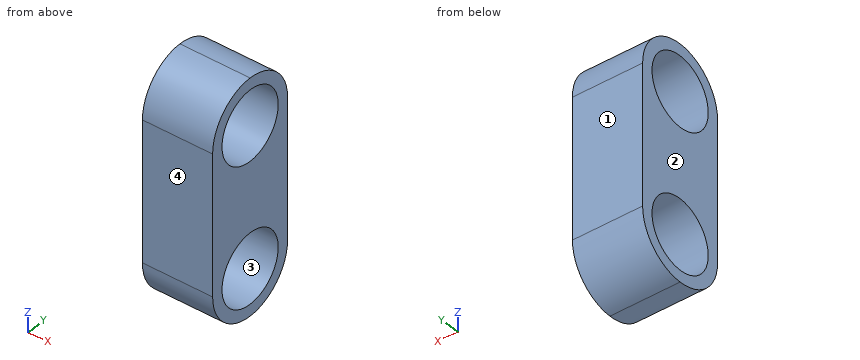
```python
from build123d import *

# Parameters (mm, degrees)
BOSS_EXTRUDE1_DEPTH = 3


with BuildPart() as part:
    # Sketch2 → Boss-Extrude1 (new body)
    with BuildSketch(Plane(origin=(0, 0, 0), x_dir=(0, 0, -1), z_dir=(1, 0, 0))):
        with BuildLine():
            Line((6, 0), (0, 0))
            ThreePointArc((0, 0), (1.414213562, -0.585786438), (2, -2))
            Line((2, -2), (4, -2))
            ThreePointArc((4, -2), (4.585786438, -0.585786438), (6, 0))
        make_face()
        with BuildLine():
            Line((4, -2), (2, -2))
            ThreePointArc((2, -2), (1.414213562, -3.414213562), (0, -4))
            Line((0, -4), (6, -4))
            ThreePointArc((6, -4), (4.585786438, -3.414213562), (4, -2))
        make_face()
        with BuildLine():
            ThreePointArc((2, -2), (1.414213562, -0.585786438), (0, 0))
            ThreePointArc((0, 0), (-1.414213562, -0.585786438), (-2, -2))
            Line((-2, -2), (-1.5, -2))
            ThreePointArc((-1.5, -2), (0, -0.5), (1.5, -2))
            Line((1.5, -2), (2, -2))
        make_face()
        with BuildLine():
            ThreePointArc((0, -4), (1.414213562, -3.414213562), (2, -2))
            Line((2, -2), (1.5, -2))
            ThreePointArc((1.5, -2), (0, -3.5), (-1.5, -2))
            Line((-1.5, -2), (-2, -2))
            ThreePointArc((-2, -2), (-1.414213562, -3.414213562), (0, -4))
        make_face()
        with BuildLine():
            ThreePointArc((8, -2), (7.414213562, -0.585786438), (6, 0))
            ThreePointArc((6, 0), (4.585786438, -0.585786438), (4, -2))
            Line((4, -2), (4.5, -2))
            ThreePointArc((4.5, -2), (6, -0.5), (7.5, -2))
            Line((7.5, -2), (8, -2))
        make_face()
        with BuildLine():
            ThreePointArc((6, -4), (7.414213562, -3.414213562), (8, -2))
            Line((8, -2), (7.5, -2))
            ThreePointArc((7.5, -2), (6, -3.5), (4.5, -2))
            Line((4.5, -2), (4, -2))
            ThreePointArc((4, -2), (4.585786438, -3.414213562), (6, -4))
        make_face()
    extrude(amount=BOSS_EXTRUDE1_DEPTH)


solid = part.part
```
Check sheet for the modelled part. Datum: model origin and axes. Units: mm. Face numbers are marked on the shaded views. Round coordinates to 2 decimals unless told otherwise and drop trailing zeros. Loops run counter-clockwise (first coordinate to the right, second up) from the corner with the lowest first, then second, coordinate; pieces in that order, holes last. Notation, with made-up numbers: (-9, 2) - (12, 2) arc R27 cw to (12, 18) - close; hole circle Ø11 at (81.25, 39.25). An arc over 180 degrees is marked (long way). Write item = value, one per line. Start each with the question number.
Q1. Depth check by flat-ended pin: P1, Ø1.5, axis at x = 2.5, y = -3.5, coming from the +Z side; P2, Ø1.5, axis at x = 2, y = -1, coming from the +Z side. Enter the tip coordinate at first touch or a pass-through.
Q2. Section check B-B (y = -3.15). Record the boundary of the cut face in (x, z).
Q3. Section check C-C (z = 1). Record the boundary of the cut face in (x, y).
Q4. Release check for a two-part mould opening along Y. For the marked faces 1, 2, 3 and 4 record: pulls with the +Y half, pulls with the -Y half, needs draft (parallel to the pull), parting line crosses it, or undercut.
Q5. Thickness scan on L1, parallel to Y at x = 1.85, z = -6; L2, parallel to Z at x = 1.15, y = -1.4; L3, parallel to Z at x = 0.1, y = -0.9. Record the ranges inside material, lowest first.
Q6. Section check A-A (x = 0.7). Record the boundary of the cut face in (y, z).
Derived:
q1.P1 = 1.85
q1.P2 = 1.98
q2.outline = (0, -7.64) - (3, -7.64) - (3, -6.96) - (0, -6.96) - close; (0, -5.04) - (3, -5.04) - (3, -0.96) - (0, -0.96) - close; (0, 0.96) - (3, 0.96) - (3, 1.64) - (0, 1.64) - close
q3.outline = (0, -3.73) - (3, -3.73) - (3, -3.12) - (0, -3.12) - close; (0, -0.88) - (3, -0.88) - (3, -0.27) - (0, -0.27) - close
q4.face_1 = pulls with the +Y half
q4.face_2 = needs draft
q4.face_3 = undercut
q4.face_4 = pulls with the -Y half
q5.L1 = -4 to -3.5, -0.5 to 0
q5.L2 = -7.91 to -7.37, -4.63 to -1.37, 1.37 to 1.91
q5.L3 = -7.67 to -7.02, -4.98 to -1.02, 1.02 to 1.67
q6.outline = (-4, -6) arc R2 ccw to (0, -6) - (0, 0) arc R2 ccw to (-4, 0) - close; hole circle Ø3 at (-2, -6); hole circle Ø3 at (-2, 0)
